from build123d import *

# Parameters (mm, degrees)
SKETCH1_R           = 1
BOSS_EXTRUDE1_DEPTH = 5
SKETCH2_R           = 1
BOSS_EXTRUDE3_DEPTH = 1
BOSS_EXTRUDE3_DRAFT = -30
CUT_EXTRUDE1_DEPTH  = 0.5
FILLET2_R           = 0.1


with BuildPart() as part:
    # Sketch1 → Boss-Extrude1 (new body)
    with BuildSketch(Plane.XY):
        Circle(SKETCH1_R)
    extrude(amount=BOSS_EXTRUDE1_DEPTH)

    # Boss-Extrude2 cone 1 section (through the dimple's axis) → Boss-Extrude2 (revolve)
    with BuildSketch(Plane(origin=(0, 0, 0), x_dir=(0, -1, 0), z_dir=(1, 0, 0))):
        Polygon((0, 0), (1, 0), (0, 1.732050808), align=None)
    revolve(axis=Axis((0, 0, 0), (0, 0, -1)))


with BuildPart() as boss_extrude3_tool:
    # Sketch2 → Boss-Extrude3 (with draft: the straight prism first)
    with BuildSketch(Plane.XY.offset(5)):
        Circle(SKETCH2_R)
    extrude(amount=BOSS_EXTRUDE3_DEPTH)
    # Boss-Extrude3: the draft: its side faces are tilted about the plane it starts from
    boss_extrude3_sides = [boss_extrude3_tool.faces().sort_by_distance(p)[0] for p in [
        (-1, 0, 5.5),
    ]]
    draft(boss_extrude3_sides, Plane.XY.offset(5), BOSS_EXTRUDE3_DRAFT)


with BuildPart() as part_1:
    add(part.part)

    # Boss-Extrude3: add boss_extrude3_tool
    add(boss_extrude3_tool.part)

    # Sketch3 → Cut-Extrude1 (cut)
    with BuildSketch(Plane.XY.offset(6)):
        with BuildLine():
            Line((-0.510620476, 1.492414353), (-0.510620476, -1.492414353))
            ThreePointArc((-0.510620476, -1.492414353), (0, -1.577350269), (0.510620476, -1.492414353))
            Line((0.510620476, -1.492414353), (0.510620476, 1.492414353))
            ThreePointArc((0.510620476, 1.492414353), (0, 1.577350269), (-0.510620476, 1.492414353))
        make_face()
    extrude(amount=-CUT_EXTRUDE1_DEPTH, mode=Mode.SUBTRACT)

    # Fillet2
    fillet2_edges = [part_1.edges().sort_by_distance(p)[0] for p in [
        (-1.577350269, 0, 6),
        (1.283250018, 0.917225852, 6),
    ]]
    fillet(fillet2_edges, radius=FILLET2_R)


solid = part_1.part
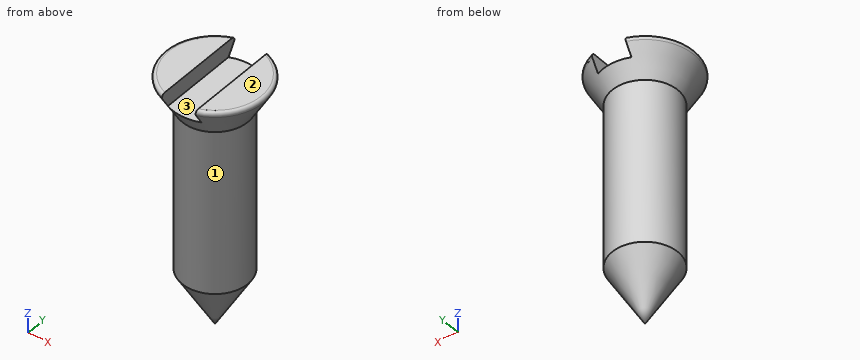
Read the model definition and answer for the solid it produces. Units are mm, in the model's axes. Face numbers are marked on the shaded views. Round coordinates to 2 decimals unless told otherwise and drop trailing zeros. Order: outer loops, then holes, each group sorted by start corner. A loop starts at its lowest first (then second) coordinate and runs counter-clockwise, first axis right, second up. Notation, with made-up numbers: (-27.75, 21.25) - (20.25, 21.25) arc R22 cw to (20.25, 44.25) - close; hole circle Ø6 at (47, -19). An arc over 180 degrees is marked (long way). Use one line per item in the form item = value. Start each with the question number.
(1) Determine the mould class of the marked faces 1, 2 and 3 for opening direction X: +X half, -X half, draft (parallel to the pull), parting line (faces both ways), or undercut.
(2) Find the intervals of material crossed by line 1 along Y through (x, z) = (-0.3, -0.5); line 2 along Y through (x, z) = (0.85, 2.5); line 3 along X through (y, z) = (-0.7, 0.5), in increasing order. Write a range as from..to.
(3) The part is cut by section B-B (z = -0.75). Give the vertices of the cut face in (x, y), then the cut area to 3 significant figures.
(4) A flat-ended cylindrical pin translates along its axis: pin 1 Ø1 at (x, z) = (0, 1) entering from -Y. Find the tip coordinate at first contact, or state that the pin passes through.
(5) The part is cut by section A-A (z = 4). Give the vertices of the cut face in (x, y).
Checked values:
q1.face_1 = parting line
q1.face_2 = draft
q1.face_3 = undercut
q2.line_1 = -0.64..0.64
q2.line_2 = -0.53..0.53
q2.line_3 = -0.71..0.71
q3.outline = circle Ø1.13 at (0, 0)
q3.area = 1.01 mm^2
q4.pin_1 = -1
q5.outline = circle Ø2 at (0, 0)
